Autodesk Inventor part; units mm, degrees
ref_plane "YZ Plane" through (0, 0, 0) normal (1, 0, 0) x (0, 1, 0)
ref_plane "XZ Plane" through (0, 0, 0) normal (0, 1, 0) x (-1, 0, 0)
ref_plane "XY Plane" through (0, 0, 0) normal (0, 0, 1) x (1, 0, 0)
sketch "Sketch1" plane through (0, 0, 0) normal (0, 0, 1) x (1, 0, 0)
  line L0 (-25, 45) -> (25, 45)
  line L1 (35, 44.3995) -> (35, -45)
  line L2 (25, -45) -> (-25, -45)
  line L3 (-35, -44.3995) -> (-35, 45)
  line L4 (-35, 45) -> (35, -45) construction
  line L5 (35, 44.3995) -> (-35, -44.3995) construction
  line L6 (-25, 55) -> (-35, 55)
  line L7 (-35, 55) -> (-35, 45)
  line L8 (-25, 45) -> (-25, 55)
  line L9 (-25, 55) -> (-35, 45) construction
  line L10 (-35, 55) -> (-25, 45) construction
  line L11 (0, 15.2738) -> (0, -11.5274)
  line L12 (-10.8069, 0) -> (18.2997, 0)
  line L13 (25, 55) -> (35, 55)
  line L14 (35, 55) -> (35, 44.3995)
  line L15 (25, 45) -> (25, 55)
  line L16 (25, 55) -> (35, 44.3995) construction
  line L17 (35, 55) -> (25, 45) construction
  line L18 (-25, -55) -> (-35, -55)
  line L19 (-35, -55) -> (-35, -44.3995)
  line L20 (-25, -45) -> (-25, -55)
  line L21 (-25, -55) -> (-35, -44.3995) construction
  line L22 (-35, -55) -> (-25, -45) construction
  line L23 (25, -55) -> (35, -55)
  line L24 (35, -55) -> (35, -45)
  line L25 (25, -45) -> (25, -55)
  line L26 (25, -55) -> (35, -45) construction
  line L27 (35, -55) -> (25, -45) construction
  point P0 (0, 0)
  point P1 (-30, 50)
  point P2 (30, 50)
  point P3 (-30, -50)
  point P4 (30, -50)
  dimension "d0" = 70
  dimension "d1" = 10
  dimension "d2" = 90
extrude "Extrusion1" add sketch "Sketch1" along normal blind 10
sketch "Sketch2" plane through (0, 0, 10) normal (0, 0, 1) x (1, 0, 0)
  circle A0 centre (0, 10.48) radius 13
  circle A1 centre (0, -19.52) radius 13
  line L0 (-25, -45) -> (25, -45)
  line L1 (-35, -55) -> (-25, -55)
  point P0 (0, 0)
  dimension "d6" = 26
  dimension "d11" = 26
  dimension "d15" = 30
  dimension "d40" = 35.48
extrude "Extrusion2" cut sketch "Sketch2" against normal blind 8
sketch "Sketch3" plane through (0, 10.48, 2) normal (0, 0, 1) x (1, 0, 0)
  circle A0 centre (0, 0) radius 5.5
  circle A1 centre (0, 0) radius 13
  point P0 (0, -10.48)
  point P1 (-9.0139, 15)
  point P2 (9.0139, 15)
  dimension "d16" = 11
extrude "Extrusion3" cut sketch "Sketch3" against normal through all contours A0
sketch "Sketch6" plane through (0, -19.52, 2) normal (0, 0, 1) x (1, 0, 0)
  circle A0 centre (0, 0) radius 5.5
  point P0 (0, 19.52)
  dimension "d19" = 11
extrude "Extrusion4" cut sketch "Sketch6" against normal blind 10
sketch "Sketch8" plane through (-25, 45, 0) normal (0, 1, 0) x (1, 0, 0)
  circle A0 centre (5, -5) radius 2.9
  line L0 (0, 0) -> (0, -10)
  line L1 (50, 0) -> (0, 0)
  circle A1 centre (45, -5) radius 2.9
  line L2 (50, 0) -> (50, -10)
  point P0 (25, 0)
  dimension "d30" = 5.8
  dimension "d31" = 5
  dimension "d32" = 5
  dimension "d33" = 5.8
  dimension "d34" = 5
  dimension "d35" = 5
extrude "Extrusion6" cut sketch "Sketch8" against normal blind 10
sketch "Sketch11" plane through (0, 0, 10) normal (0, 0, 1) x (1, 0, 0)
  line L0 (-35, 55) -> (-35, -55)
  line L1 (-25, 55) -> (-35, 55)
  line L2 (0, 0) -> (0, 27.2927)
  line L3 (0, 0) -> (14.8331, 0)
  circle A0 centre (-30, -50) radius 2.1
  circle A1 centre (30, -50) radius 2.1
  line L4 (-35, -55) -> (-25, -55)
  line L5 (25, -45) -> (25, -55)
  line L6 (25, -55) -> (35, -55)
  point P0 (30, -55)
  dimension "d54" = 4.2
  dimension "d55" = 5
  dimension "d56" = 5
  dimension "d57" = 4.2
  dimension "d58" = 5
  dimension "d59" = 5
extrude "Extrusion9" cut sketch "Sketch11" against normal through all
sketch "Sketch7" plane through (0, -48, 10) normal (0, 0, -1) x (-1, 0, 0)
  circle A0 centre (0, 22.5) radius 1.6
  circle A1 centre (-22.5, 0) radius 1.6
  circle A2 centre (0, -22.5) radius 1.6
  circle A3 centre (22.5, 0) radius 1.6
  point P0 (0, 48)
  point P1 (0, 0)
  dimension "d22" = 3.2
  dimension "d25" = 360
  dimension "d27" = 45
equation "\"d33\" = d30"
equation "\"d57\" = d54"
equation "\"d58\" = d55"
properties part number "gearbox_side1" material "PMMA Plastic"
Build history of the part. All positions in model axes, mm. A direction names the side the tool comes from. Give positions to 0.01 mm unless a question says otherwise; leave off trailing zeros. Loops run counter-clockwise (first coordinate to the right, second up) from the corner with the lowest first, then second, coordinate; pieces in that order, holes last. Notation, with made-up numbers: (-12, 85.5) - (-5, 85.5) arc R24 cw to (-5, 104.5) - close; hole circle Ø10 at (35.5, 37.25). An arc over 180 degrees is marked (long way). Use a Markdown table: item, result.
(1) Band-saw the part on D-D (x = 30). Give the cut face in (y, z), and give its area (3 significant figures).
Taken from the geometry:
| item | result |
|---|---|
| outline | (-55, 0) - (-52.1, 0) - (-52.1, 10) - (-55, 10) - close; (-47.9, 0) - (55, 0) - (55, 10) - (-47.9, 10) - close |
| area | 1,060 mm2 |
(2) Band-saw the part on C-C (y = -19.52). Give the cut face in (x, z), and give its area (3 significant figures).
Taken from the geometry:
| item | result |
|---|---|
| outline | (-35, 0) - (-5.5, 0) - (-5.5, 2) - (-13, 2) - (-13, 10) - (-35, 10) - close; (5.5, 0) - (35, 0) - (35, 10) - (13, 10) - (13, 2) - (5.5, 2) - close |
| area | 470 mm2 |
(3) Pull direction Z, two halves, no side cores. Call faces 6 (the face through (-30, -55, 5)), 7 (the face through (-16, 1, 10)), 8 (the face through (-22.9, 40.1, 4.9)): +Z half, -Z half, draft (parallel to the pull), parting line (faces both ways), or undercut.
Taken from the geometry:
| item | result |
|---|---|
| face 6 | draft |
| face 7 | +Z half |
| face 8 | undercut |
(4) Drop flat-ended pins along their axis: pin 1 Ø4 at (x, y) = (-30, -50) entering from +Z; pin 2 Ø8 at (x, y) = (-5, -23.5) entering from +Z; pin 3 Ø12 at (x, y) = (3, 31) entering from -Z; pin 4 Ø3 at (x, z) = (-13, 3.5) entering from -Y. Give the stop position or say it passes through.
Taken from the geometry:
| item | result |
|---|---|
| pin 1 | through |
| pin 2 | z = 2 |
| pin 3 | z = 0 |
| pin 4 | y = -45 |
(5) Which spindle directions (+Z, -Z, +X, -X, +Y, -Y) get a long thin tool onto all of the face, cutting with end or side? Do faces 1 (the face through (17.1, 40.1, 4.9)), 2 (the face through (25, -50, 5)), 3 (the face through (6, 11, 2)), 4 (the face through (25, 50, 5)), 5 (the face through (35, 1, 5)). Say none if no direction does.
Taken from the geometry:
| item | result |
|---|---|
| face 1 | +Y |
| face 2 | +Z, -Z, -Y |
| face 3 | +Z |
| face 4 | +Z, -Z, +Y |
| face 5 | +Z, -Z, +X, +Y, -Y |
(6) Wall check: line 1 along Y through (x, z) = (0, 1.45); line 2 along X through (y, z) = (37.5, 5); line 3 along Z through (x, y) = (-20, 37.25). Give the ranges that are in metal, low to high.
Taken from the geometry:
| item | result |
|---|---|
| line 1 | -45 to -25.02, -14.02 to 4.98, 15.98 to 45 |
| line 2 | -35 to -22.9, -17.1 to 17.1, 22.9 to 35 |
| line 3 | 0 to 2.1, 7.9 to 10 |
(7) Band-saw the part on A-A (z = 5). Give the cut face in (x, y), and give its area (3 significant figures).
Taken from the geometry:
| item | result |
|---|---|
| outline | (-35, -55) - (-25, -55) - (-25, -45) - (25, -45) - (25, -55) - (35, -55) - (35, 55) - (25, 55) - (25, 45) - (22.9, 45) - (22.9, 35) - (17.1, 35) - (17.1, 45) - (-17.1, 45) - (-17.1, 35) - (-22.9, 35) - (-22.9, 45) - (-25, 45) - (-25, 55) - (-35, 55) - close; hole circle Ø4.2 at (-30, -50); hole circle Ø26 at (0, -19.52); hole circle Ø26 at (0, 10.48); hole circle Ø4.2 at (30, -50) |
| area | 5,490 mm2 |
(8) Band-saw the part on B-B (x = 0). Give the cut face in (y, z).
Taken from the geometry:
| item | result |
|---|---|
| outline | (-45, 0) - (-25.02, 0) - (-25.02, 2) - (-32.52, 2) - (-32.52, 10) - (-45, 10) - close; (-14.02, 0) - (4.98, 0) - (4.98, 2) - (-2.52, 2) - (-2.52, 10) - (-6.52, 10) - (-6.52, 2) - (-14.02, 2) - close; (15.98, 0) - (45, 0) - (45, 10) - (23.48, 10) - (23.48, 2) - (15.98, 2) - close |
